Could you check a few things on this model? Use its own coordinates, in mm. Face numbers are marked on the shaded views. A direction names the side the tool comes from. Round coordinates to 2 decimals unless told otherwise and drop trailing zeros. Write each loop counter-clockwise with the first axis right and the second up, starting at its lowest first coordinate (ties: lowest second). Pieces come first, ordered by that corner, then holes. Notation, with made-up numbers: (43, -7.75) - (56, -7.75) arc R8 cw to (56, 4.25) - close; hole circle Ø8 at (-5, -33). An arc over 180 degrees is marked (long way). Put each result on its own line as item: value.
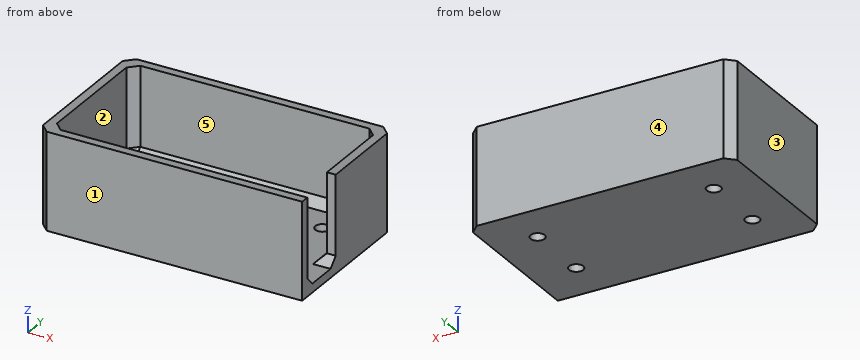
Autodesk Inventor part; units mm, degrees
ref_plane "YZ Plane" through (0, 0, 0) normal (1, 0, 0) x (0, 1, 0)
ref_plane "XZ Plane" through (0, 0, 0) normal (0, 1, 0) x (-1, 0, 0)
ref_plane "XY Plane" through (0, 0, 0) normal (0, 0, 1) x (1, 0, 0)
sketch "スケッチ1" plane through (0, 0, 0) normal (0, 0, 1) x (1, 0, 0)
  line L0 (0, 0) -> (60, 0)
  line L1 (60, 0) -> (60, 35)
  line L2 (60, 35) -> (0, 35)
  line L3 (0, 35) -> (0, 0)
  dimension "d0" = 60
  dimension "d1" = 35
extrude "押し出し1" add sketch "スケッチ1" along normal blind 2
sketch "スケッチ2" plane through (0, 0, 2) normal (0, 0, 1) x (1, 0, 0)
  line L0 (60, 35) -> (0, 35)
  line L1 (2, 33) -> (2, 2)
  line L2 (0, 35) -> (0, 0)
  line L3 (58, 33) -> (58, 13.0563)
  line L4 (60, 0) -> (60, 35)
  line L5 (2, 33) -> (58, 33)
  line L6 (2, 2) -> (58, 2)
  line L7 (0, 0) -> (60, 0)
  line L8 (58, 13.0563) -> (60, 13.0563)
  line L9 (60, 2) -> (58, 2)
  line L10 (0, 35) -> (60, 35)
  line L11 (60, 0) -> (0, 0)
  line L12 (0, 0) -> (0, 35)
  line L13 (60, 13.0563) -> (58, 13.0563)
  line L14 (60, 2) -> (2, 2)
  line L15 (60, 35) -> (60, 13.0563)
  line L16 (60, 2) -> (60, 0)
  dimension "d4" = 2
  dimension "d5" = 2
  dimension "d6" = 2
extrude "押し出し3" add sketch "スケッチ2" along normal blind 20 contours L4 L8 L3 L5 L1 L6 L9 L7 L2 L0
sketch "スケッチ3" plane through (0, 0, 2) normal (0, 0, 1) x (1, 0, 0)
  circle A0 centre (10, 25) radius 1.6
  line L0 (60, 35) -> (0, 35)
  line L1 (0, 35) -> (0, 0)
  circle A1 centre (50, 25) radius 1.6
  circle A2 centre (10, 10) radius 1.6
  circle A3 centre (50, 10) radius 1.6
  dimension "d12" = 3.2
  dimension "d13" = 10
  dimension "d14" = 10
  dimension "d15" = 3.2
  dimension "d16" = 3.2
  dimension "d17" = 3.2
extrude "押し出し4" cut sketch "スケッチ3" against normal blind 2
chamfer "面取り1" distance 2 angle 45 7 edges at (2, 17.5, 2) (30, 33, 2) (31, 2, 2) (2, 2, 12) (2, 33, 12) (60, 35, 11) (58, 23.0282, 2)
chamfer "面取り2" distance 2 angle 45 2 edges at (59, 13.0563, 2) (58, 33, 13)
chamfer "面取り3" distance 2 angle 45 2 edges at (0, 0, 11) (0, 35, 11)
properties part number "LiFeCase"
(1) Imagine slicing it at B-B, the plane x = 50. List the corners of the cut face in (y, z) for me, then the cut area to 3 significant figures.
Values found:
outline: (0, 0) - (8.4, 0) - (8.4, 2) - (4, 2) - (2, 4) - (2, 22) - (0, 22) - close; (11.6, 0) - (23.4, 0) - (23.4, 2) - (11.6, 2) - close; (26.6, 0) - (35, 0) - (35, 22) - (33, 22) - (33, 4) - (31, 2) - (26.6, 2) - close
area: 141 mm^2
(2) Imagine slicing it at C-C, the plane z = 16.75. List the corners of the cut face in (x, y) for me, then the cut area to 3 significant figures.
Values found:
outline: (0, 2) - (2, 0) - (60, 0) - (60, 2) - (4, 2) - (2, 4) - (2, 31) - (4, 33) - (56, 33) - (58, 31) - (58, 13.06) - (60, 13.06) - (60, 33) - (58, 35) - (2, 35) - (0, 33) - close
area: 342 mm^2
(3) For the marked faces 4 and 5, which set-ups out of +Z, -Z, +X, -X, +Y, -Y let a thin tool reach every point of the face, with its end or its side?
Values found:
face 4: +Z, -Z, +X, -X, +Y
face 5: +Z
(4) Imagine slicing it at A-A, the plane y = 25. List the corners of the cut face in (x, z) for me, then the cut area to 3 significant figures.
Values found:
outline: (0, 0) - (8.4, 0) - (8.4, 2) - (4, 2) - (2, 4) - (2, 22) - (0, 22) - close; (11.6, 0) - (48.4, 0) - (48.4, 2) - (11.6, 2) - close; (51.6, 0) - (60, 0) - (60, 22) - (58, 22) - (58, 4) - (56, 2) - (51.6, 2) - close
area: 191 mm^2
(5) I'm going to push flat-ended pins straight in: pin 1 (2 mm diameter, centred on y = 17.5, z = 11.5, fed in from -X); pin 2 (8 mm diameter, centred on x = 39, y = 19.5, fed in from +Z); pin 3 (8 mm diameter, centred on x = 19, y = 28.5, fed in from +Z); pin 4 (6 mm diameter, centred on x = 38, y = 6, fed in from +Z). Where does each tip first touch, or does it pass through?
Values found:
pin 1: stops at x = 0
pin 2: stops at z = 2
pin 3: stops at z = 3.5
pin 4: stops at z = 3
(6) Please list where these lines run through material, in increasing order: probe 1 along Y at (x, z) = (50, 0.75); probe 2 along Y at (x, z) = (33.5, 16.75); probe 3 along X at (y, z) = (20.5, 5). Write a range as from..to.
Values found:
probe 1: y = 0..8.4, 11.6..23.4, 26.6..35
probe 2: y = 0..2, 33..35
probe 3: x = 0..2, 58..60
(7) Imagine slicing it at D-D, the plane x = 7.5. List the corners of the cut face in (y, z) for me.
Values found:
outline: (0, 0) - (35, 0) - (35, 22) - (33, 22) - (33, 4) - (31, 2) - (4, 2) - (2, 4) - (2, 22) - (0, 22) - close
(8) If we mould it in two halves opening along Y, with no side actions, what happens to the marked faces 1, 2 and 3? For each: pulls with the +Y half, pulls with the -Y half, needs draft (parallel to the pull), parting line crosses it, or undercut.
Values found:
face 1: pulls with the -Y half
face 2: undercut
face 3: needs draft
